Part model, mm, in its own coordinate system. A direction names the side the tool comes from. Give positions to 0.01 mm unless a question says otherwise; leave off trailing zeros. Order: outer loops, then holes, each group sorted by start corner. A loop starts at its lowest first (then second) coordinate and runs counter-clockwise, first axis right, second up. Notation, with made-up numbers: (66.5, -22.5) - (104.5, -22.5) arc R32 ccw to (104.5, 16.5) - close; hole circle Ø9 at (32, 7). An arc over 180 degrees is marked (long way). Use one line per item in the form item = value. Start each with the question number.
1. Pull direction X, two halves, no side cores. Call faces 3 (the face through (-16, 0, 4)), 4 (the face through (13.265, 12.898, 6.409)), 5 (the face through (-12.898, 13.265, 6.409)): +X half, -X half, draft (parallel to the pull), parting line (faces both ways), or undercut.
2. Band-saw the part on B-B, the plane y = -18.5. List the corners of the cut face in (x, z), plus the area to 3 significant figures.
3. Tool access for faces 1 (the face through (18, -3, 8.6)), 2 (the face through (21, 0, 4)): list every direction of +Z, -Z, +X, -X, +Y, -Y with a clear straight run to the whole face (end or side of a thin tool).
4. Band-saw the part on D-D, the plane z = 4.5. List the corners of the cut face in (x, y), plus the area to 3 significant figures.
5. Drill centre lines: line 1 (Y direction, x = 0.5, z = 12.25); line 2 (X direction, y = -15, z = 9.25); line 3 (X direction, y = 16.5, z = 1.75). Where is each one in solid material? Low to high.
6. Pin check, flat tips, straight feed: P1, Ø7, axis at x = 18.5, y = 0, coming from the +Z side; P2, Ø3, axis at y = -2.5, z = 6, coming from the +X side; P3, Ø1, axis at y = 14.5, z = 10, coming from the +X side; P4, Ø4.5, axis at x = 18.5, y = 0, coming from the -Z side. Stop position of each tip, or through.
7. Band-saw the part on A-A, the plane z = 11.25. List the corners of the cut face in (x, y).
from build123d import *

# Parameters (mm, degrees)
SKETCH_1_R          = 2.5
SKETCH_1_R_2        = 4
EXTRUDE_1_DEPTH     = 13
SKETCH_2_R          = 4
CUT_EXTRUDE_1_DEPTH = 4.4


with BuildPart() as part:
    # 草图1 → 凸台-拉伸1 (new body)
    with BuildSketch(Plane.XY):
        Polygon((0, 26.162950904), (-26.162950904, 0), (0, -26.162950904), (26.162950904, 0), align=None)
        with Locations(Location((18.5, 0, 0), (0, 0, 180))):
            Circle(SKETCH_1_R, mode=Mode.SUBTRACT)
        with Locations(Location((0, -18.5, 0), (0, 0, 180))):
            Circle(SKETCH_1_R, mode=Mode.SUBTRACT)
        with Locations(Location((-18.5, 0, 0), (0, 0, 180))):
            Circle(SKETCH_1_R, mode=Mode.SUBTRACT)
        with Locations(Location((0, 18.5, 0), (0, 0, 180))):
            Circle(SKETCH_1_R, mode=Mode.SUBTRACT)
        with Locations(Location((0, 0, 0), (0, 0, 180))):
            Circle(SKETCH_1_R_2, mode=Mode.SUBTRACT)
    extrude(amount=EXTRUDE_1_DEPTH)

    # 草图2 → 切除-拉伸1 (cut)
    with BuildSketch(Plane.XY.offset(13)):
        with Locations((18.5, 0)):
            Circle(SKETCH_2_R)
        with Locations((0, -18.5)):
            Circle(SKETCH_2_R)
        with Locations((-18.5, 0)):
            Circle(SKETCH_2_R)
        with Locations((0, 18.5)):
            Circle(SKETCH_2_R)
    extrude(amount=-CUT_EXTRUDE_1_DEPTH, mode=Mode.SUBTRACT)


solid = part.part
From the geometry:
q1.face_3 = undercut
q1.face_4 = +X half
q1.face_5 = -X half
q2.outline = (-7.66, 0) - (-2.5, 0) - (-2.5, 8.6) - (-4, 8.6) - (-4, 13) - (-7.66, 13) - close; (2.5, 0) - (7.66, 0) - (7.66, 13) - (4, 13) - (4, 8.6) - (2.5, 8.6) - close
q2.area = 121 mm²
q3.face_1 = +Z
q3.face_2 = +Z, -Z
q4.outline = (-26.16, 0) - (0, -26.16) - (26.16, 0) - (0, 26.16) - close; hole circle Ø5 at (-18.5, 0); hole circle Ø8 at (0, 0); hole circle Ø5 at (0, -18.5); hole circle Ø5 at (0, 18.5); hole circle Ø5 at (18.5, 0)
q4.area = 1,240 mm²
q5.line_1 = -25.66 to -22.47, -14.53 to -3.97, 3.97 to 14.53, 22.47 to 25.66
q5.line_2 = -11.16 to -1.94, 1.94 to 11.16
q5.line_3 = -9.66 to -1.5, 1.5 to 9.66
q6.P1 = 8.6
q6.P2 = 25.16
q6.P3 = 12.16
q6.P4 = through
q7.outline = (-26.16, 0) - (0, -26.16) - (26.16, 0) - (0, 26.16) - close; hole circle Ø8 at (-18.5, 0); hole circle Ø8 at (0, -18.5); hole circle Ø8 at (0, 0); hole circle Ø8 at (0, 18.5); hole circle Ø8 at (18.5, 0)
